The model under review builds one solid part; all positions refer to its coordinate system, in mm. Face numbers are marked on the shaded views. Give positions to 0.01 mm unless a question says otherwise; leave off trailing zeros. Order: outer loops, then holes, each group sorted by start corner. A loop starts at its lowest first (then second) coordinate and runs counter-clockwise, first axis right, second up. Notation, with made-up numbers: (34.25, 88.5) - (68.25, 88.5) arc R18 ccw to (68.25, 99.5) - close; hole circle Ø3 at (82.5, 80.25). An arc over 180 degrees is marked (long way). Write item = value, one per line. Start each with the question number.
1. Wall thickness on probe 1 along Z at (x, y) = (0, 26); probe 2 along Z at (x, y) = (0, 26.15); probe 3 along X at (y, z) = (25.85, 0): over which ranges is each line inside the solid? List them lowest first.
2. Mouldability with a two-part tool opening along Z and no side actions: class the marked faces 1, 2 and 3 as pulls with the +Z half, pulls with the -Z half, needs draft (parallel to the pull), parting line crosses it, or undercut.
3. We need section A-A, the plane y = 8. Give the boundary of the cut face in (x, z).
4. For P1, Ø6, axis at y = 4.5, z = -17, coming from the -X side; P2, Ø4, axis at y = 25, z = -3, coming from the -X side; P3, Ø1, axis at y = 5.5, z = -17, coming from the -X side, all flat-tipped, find the tip position at first contact; note any pin that passes through.
5. We need section B-B, the plane y = 2. Give the boundary of the cut face in (x, z), and give its area (3 significant figures).
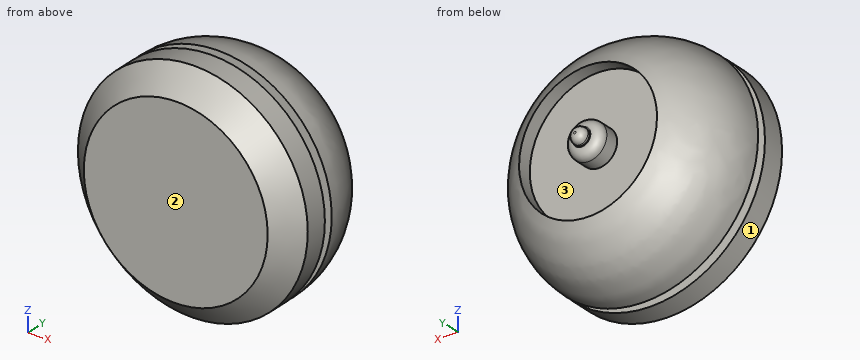
Autodesk Inventor part; units mm, degrees
ref_plane "Work Plane1" through (0, 12, 0) normal (0, 1, 0) x (-1, 0, 0)
ref_plane "YZ Plane" through (0, 0, 0) normal (1, 0, 0) x (0, 1, 0)
ref_plane "XY Plane" through (0, 0, 0) normal (0, 0, 1) x (1, 0, 0)
sketch "Sketch1" plane through (0, 0, 0) normal (0, 1, 0) x (-1, 0, 0)
  circle A0 centre (0, 0) radius 25
  dimension "d0" = 50
extrude "Extrusion1" add sketch "Sketch1" along normal blind 30
fillet "Fillet1" radius 18 1 edges at (25, 30, 0)
chamfer "Chamfer1" distance 5 angle 45 1 edges at (25, 0, 0)
sketch "Sketch2" plane through (0, 30, 0) normal (0, 1, 0) x (1, 0, 0)
  line L0 (0, 0) -> (6.5883, 0)
  line L1 (6.5883, 0) -> (-7, 0)
  circle A0 centre (0, 0) radius 7
  circle A1 centre (0, 0) radius 6.5883
  circle A2 centre (0, 0) radius 25
  circle A3 centre (0, 0) radius 15
  dimension "d7" = 30
extrude "Extrusion2" cut sketch "Sketch2" against normal blind 5 contours L1 A1 L0 | L0 A1 L1 | A0 | A3
sketch "Sketch3" plane through (0, 25, 0) normal (0, 1, 0) x (1, 0, 0)
  circle A0 centre (0, 0) radius 4
  dimension "d10" = 8
extrude "Extrusion3" add sketch "Sketch3" along normal blind 5
fillet "Fillet2" radius 2 1 edges at (-4, 30, 0)
ref_plane "Work Plane1" through (0, 12, 0) normal (0, 1, 0) x (-1, 0, 0)
sketch "Sketch4" plane through (0, 12, 0) normal (0, 1, 0) x (-1, 0, 0)
  circle A0 centre (0, 0) radius 4
  circle A1 centre (0, 0) radius 25
  circle A2 centre (0, 0) radius 2
  circle A3 centre (0, 0) radius 15
  dimension "d21" = 30
sketch "Sketch5" plane through (0, 30, 0) normal (0, 1, 0) x (1, 0, 0)
  circle A0 centre (0, 0) radius 2
  circle A1 centre (0, 0) radius 1.75
  dimension "d17" = 3.5
extrude "Extrusion5" add sketch "Sketch5" along normal blind 2 contours A1
fillet "Fillet3" radius 1.5 1 edges at (-1.75, 32, 0)
extrude "Extrusion6" cut sketch "Sketch4" against normal blind 2 contours A1
properties part number "camera"
Model answer:
q1.probe_1 = -18.31 to -15, -4 to 4, 15 to 18.31
q1.probe_2 = -18.13 to -15, -4 to 4, 15 to 18.13
q1.probe_3 = -18.5 to -15, -4 to 4, 15 to 18.5
q2.face_1 = parting line crosses it
q2.face_2 = needs draft
q2.face_3 = undercut
q3.outline = circle Ø50 at (0, 0)
q4.P1 = -20.68
q4.P2 = -21.06
q4.P3 = -18.78
q5.outline = circle Ø44 at (0, 0)
q5.area = 1,520 mm2
